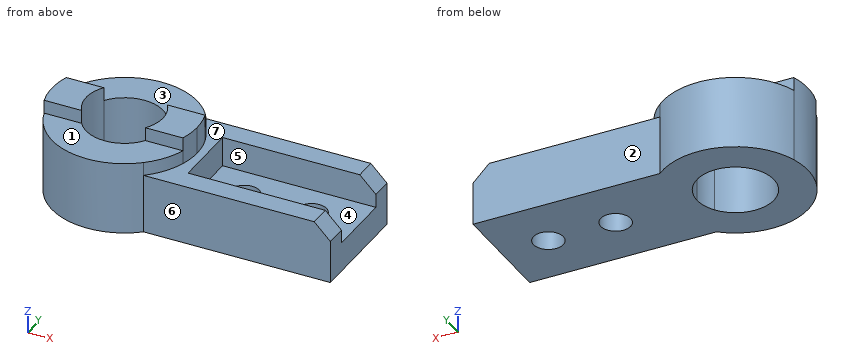
from build123d import *

# Parameters (mm, degrees)
F1_DEPTH = 54
F2_DEPTH = 64
F3_DEPTH = 44
F0_W     = 114
F0_H     = 50
F0_R     = 11.1
F4_DEPTH = 22
F5_SIZE2 = 12
F5_SIZE  = 12


with BuildPart() as f1:
    # F0 (on Top) → F1 (new body)
    with BuildSketch(Plane.XY):
        with BuildLine():
            Line((23.675528, 16), (51.575188, 16))
            ThreePointArc((51.575188, 16), (45.124741, 29.660711), (35.142567, 41))
            ThreePointArc((35.142567, 41), (-14.958535, 51.886821), (-51.575188, 16))
            Line((-51.575188, 16), (-23.675528, 16))
            ThreePointArc((-23.675528, 16), (0, 28.575), (23.675528, 16))
        make_face()
        with BuildLine():
            ThreePointArc((35.142567, -41), (45.124741, -29.660711), (51.575188, -16))
            Line((51.575188, -16), (23.675528, -16))
            ThreePointArc((23.675528, -16), (0, -28.575), (-23.675528, -16))
            Line((-23.675528, -16), (-51.575188, -16))
            ThreePointArc((-51.575188, -16), (-14.958535, -51.886821), (35.142567, -41))
        make_face()
    extrude(amount=F1_DEPTH)



with BuildPart() as f2:
    # F0 (on Top) → F2 (new body)
    with BuildSketch(Plane.XY):
        with BuildLine():
            Line((-23.675528, 16), (-51.575188, 16))
            ThreePointArc((-51.575188, 16), (-54, 0), (-51.575188, -16))
            Line((-51.575188, -16), (-23.675528, -16))
            ThreePointArc((-23.675528, -16), (-28.575, 0), (-23.675528, 16))
        make_face()
        with BuildLine():
            ThreePointArc((51.575188, -16), (53.390356, -8.091349), (54, 0))
            ThreePointArc((54, 0), (53.390356, 8.091349), (51.575188, 16))
            Line((51.575188, 16), (23.675528, 16))
            ThreePointArc((23.675528, 16), (27.322691, 8.366672), (28.575, 0))
            ThreePointArc((28.575, 0), (27.322691, -8.366672), (23.675528, -16))
            Line((23.675528, -16), (51.575188, -16))
        make_face()
    extrude(amount=F2_DEPTH)


with BuildPart() as f1_1:
    add(f1.part)

    add(f2.part)  # F3 merges F2
    # F0 (on Top) → F3 (join)
    with BuildSketch(Plane.XY):
        with BuildLine():
            ThreePointArc((51.575188, 16), (53.390356, 8.091349), (54, 0))
            ThreePointArc((54, 0), (53.390356, -8.091349), (51.575188, -16))
            ThreePointArc((51.575188, -16), (45.124741, -29.660711), (35.142567, -41))
            Line((35.142567, -41), (174, -41))
            Line((174, -41), (174, -25))
            Line((174, -25), (60, -25))
            Line((60, -25), (60, 25))
            Line((60, 25), (174, 25))
            Line((174, 25), (174, 41))
            Line((174, 41), (35.142567, 41))
            ThreePointArc((35.142567, 41), (45.124741, 29.660711), (51.575188, 16))
        make_face()
    extrude(amount=F3_DEPTH)

    # F0 (on Top) → F4 (join)
    with BuildSketch(Plane.XY):
        with Locations((117, 0)):
            Rectangle(F0_W, F0_H)
        with Locations((89, 0)):
            Circle(F0_R, mode=Mode.SUBTRACT)
        with Locations((139, 0)):
            Circle(F0_R, mode=Mode.SUBTRACT)
    extrude(amount=F4_DEPTH)

    # F5
    f5_edges = [f1_1.edges().sort_by_distance(p)[0] for p in [
        (174, -33, 44),
        (174, 33, 44),
    ]]
    chamfer(f5_edges, length=F5_SIZE, length2=F5_SIZE2)


solid = f1_1.part
Part model, mm, in its own coordinate system. Face numbers are marked on the shaded views. A direction names the side the tool comes from. Give positions to 0.01 mm unless a question says otherwise; leave off trailing zeros. Order: outer loops, then holes, each group sorted by start corner. A loop starts at its lowest first (then second) coordinate and runs counter-clockwise, first axis right, second up. Notation, with made-up numbers: (-27.5, 46.25) - (1.5, 46.25) arc R11 cw to (1.5, 52.25) - close; hole circle Ø6 at (83.25, 27). An arc over 180 degrees is marked (long way). Use a Markdown table: item, result.
1) Flat gauge pins, fed straight in: P1, Ø11, axis at x = -40, z = 58.5, coming from the +Y side; P2, Ø11.5, axis at x = 3.5, y = 44.5, coming from the +Z side; P3, Ø3, axis at x = -36, z = 59, coming from the -Y side; P4, Ø5, axis at x = 127, z = 47.5, coming from the +Y side. Where does each tip first touch, or does it go through?
Checked values:
| item | result |
|---|---|
| P1 | y = 39.48 |
| P2 | z = 54 |
| P3 | y = -16 |
| P4 | through |
2) Probe L1, parallel to Y at x = -1, z = 11; L2, parallel to X at y = -3.5, z = 8; L3, parallel to Y at x = 94, z = 22.5. List the from-to ranges inside material, lowest first. Write a range as from..to.
Checked values:
| item | result |
|---|---|
| L1 | -53.99..-28.56, 28.56..53.99 |
| L2 | -53.89..-28.36, 28.36..78.47, 99.53..128.47, 149.53..174 |
| L3 | -41..-25, 25..41 |
3) Saw through at A-A on x = 139. List the corners of the cut face in (y, z), plus the area to 3 significant figures.
Checked values:
| item | result |
|---|---|
| outline | (-41, 0) - (-11.1, 0) - (-11.1, 22) - (-25, 22) - (-25, 44) - (-41, 44) - close; (11.1, 0) - (41, 0) - (41, 44) - (25, 44) - (25, 22) - (11.1, 22) - close |
| area | 2,020 mm² |
4) Saw through at C-C on z = 26. List the corners of the cut face in (x, y) (3 decimals).
Checked values:
| item | result |
|---|---|
| outline | (-51.575, -16) arc R54 ccw to (35.143, -41) - (174, -41) - (174, -25) - (60, -25) - (60, 25) - (174, 25) - (174, 41) - (35.143, 41) arc R54 ccw to (-51.575, 16) arc R54 ccw to start; hole (23.676, -16) arc R28.575 ccw to (28.575, 0) arc R28.575 ccw to (23.676, 16) arc R28.575 ccw (long way) to start |
5) Two-plate mould, pull along Y, no slides. Class the marked faces 5, 6 and 7: +Y half, -Y half, draft (parallel to the pull), parting line (faces both ways), or undercut.
Checked values:
| item | result |
|---|---|
| face 5 | undercut |
| face 6 | -Y half |
| face 7 | draft |
6) Saw through at B-B on z = 59.5. List the corners of the cut face in (x, y) (3 decimals), plus the area to 3 significant figures.
Checked values:
| item | result |
|---|---|
| outline | (-51.575, -16) - (-23.676, -16) arc R28.575 cw to (-23.676, 16) - (-51.575, 16) arc R54 ccw to start; (23.676, -16) - (51.575, -16) arc R54 ccw to (54, 0) arc R54 ccw to (51.575, 16) - (23.676, 16) arc R28.575 cw to (28.575, 0) arc R28.575 cw to start |
| area | 1,680 mm² |
7) Saw through at D-D on x = 75. List the corners of the cut face in (y, z).
Checked values:
| item | result |
|---|---|
| outline | (-41, 0) - (41, 0) - (41, 44) - (25, 44) - (25, 22) - (-25, 22) - (-25, 44) - (-41, 44) - close |
8) 3-axis set-ups, long thin cutter, end or side, ignore diameter. For the marked faces 1, 2, 3 and 4: which of +Z, -Z, +X, -X, +Y, -Y reach the whole face in a straight line?
Checked values:
| item | result |
|---|---|
| face 1 | +Z, +X, -X, -Y |
| face 2 | +Z, -Z, +X, +Y |
| face 3 | +Z, +X, -X, +Y |
| face 4 | +Z, +X |
